Verification items for the finished model (mm, model axes). A direction names the side the tool comes from. Give positions to 0.01 mm unless a question says otherwise; leave off trailing zeros. Write each loop counter-clockwise with the first axis right and the second up, starting at its lowest first coordinate (ties: lowest second). Pieces come first, ordered by that corner, then holes. Notation, with made-up numbers: (-0.5, 3.25) -> (31.5, 3.25) arc R34 cw to (31.5, 40.25) -> close; hole circle Ø10 at (75.5, 13). An arc over 180 degrees is marked (long way). Answer as CSV lines item,"result". Start each with the question number.
1) Sectioned sample at D-D on y = 15.5. Record the cut outline in (x, z), and give its area (3 significant figures).
2) Gauge pin test, flat ends, axial feed: pin 1 Ø2 at (x, z) = (4, 9) entering from -Y; pin 2 Ø1.8 at (y, z) = (18, 6) entering from +X; pin 3 Ø1 at (x, z) = (1, 8.5) entering from -Y. Record the tip position at first contact, or that the pin passes through.
3) Sectioned sample at C-C on z = 8.75. Record the cut outline in (x, y) (3 decimals), and give its area (3 significant figures).
4) Sectioned sample at B-B on y = 34. Record the cut outline in (x, z).
5) Tool access check on faces 1 (the flat face through (3, 15, 5)), 2 (the flat face through (0, 5, 5)), 3 (the cylindrical face through (1.1, 38.3, 9)), 4 (the flat face through (0, 25, 5)). Record the directions out of +Z, -Z, +X, -X, +Y, -Y that give a thin tool (end or side, any length) a straight path to the whole face; none if there is none.
6) Mould release check, pull along Z, two halves, no side actions. Record for faces 5 (the flat face through (-3, 15, 5)), 6 (the flat face through (5, 20, 9)), 7 (the flat face through (-3.4, 20.4, 2)), 8 (the flat face through (0, 20, 0)): released by +Z, released by -Z, zero draft, split by the parting line, or undercut.
7) Material ranges on L1, parallel to Y at x = 0, z = 9.65 (3 decimals); L2, parallel to X at y = 0, z = 8.85; L3, parallel to Z at x = -3.5, y = 12, recorded low to high.
8) Sectioned sample at A-A on x = 0. Record the cut outline in (y, z) (3 decimals), and give its area (3 significant figures).
Autodesk Inventor part; units mm, degrees
ref_plane "YZ Plane" through (0, 0, 0) normal (1, 0, 0) x (0, 1, 0)
ref_plane "XZ Plane" through (0, 0, 0) normal (0, 1, 0) x (-1, 0, 0)
ref_plane "XY Plane" through (0, 0, 0) normal (0, 0, 1) x (1, 0, 0)
sketch "Sketch1" plane through (0, 0, 0) normal (0, 0, 1) x (1, 0, 0)
  circle A0 centre (0, 0) radius 2.05
  arc A1 (-5, 0) -> (5, 0) centre (0, 0) ccw
  circle A2 centre (0, 40) radius 2.025
  arc A3 (5, 40) -> (-5, 40) centre (0, 40) ccw
  line L0 (-5, 40) -> (-5, 0)
  line L1 (5, 40) -> (5, 0)
  line L2 (0, 0) -> (0, 2.05)
  line L3 (0, 37.975) -> (0, 40)
  dimension "d0" = 4.1
  dimension "d3" = 4.05
  dimension "d1" = 10
  dimension "d2" = 40
  dimension "d4" = 10
extrude "Extrusion1" add sketch "Sketch1" along normal blind 10
shell "Shell1" thickness 2 removed faces 4 at (3.9972, 43.0037, 6.6667) at (-4.9838, -0.4023, 6.6667) at (-5, 13.3333, 3.3333) at (5, 26.6667, 3.3333)
sketch "Sketch2" plane through (0, 40, 8) normal (0, 0, -1) x (-1, 0, 0)
  line L0 (-3, -35) -> (3, -35)
  line L1 (3, -35) -> (3, -15)
  line L2 (3, -15) -> (-3, -15)
  line L3 (-3, -15) -> (-3, -35)
  circle A0 centre (0, 0) radius 2.025
  point P0 (0, -40)
  dimension "d13" = 6
  dimension "d14" = 20
  dimension "d18" = 5
extrude "Extrusion2" add sketch "Sketch2" along normal blind 6 contours L3 L2 L1 L0
delete faces "Delete Face1" heal yes whole lump no faces at (4.0369, 0.3259, 4)
delete faces "Delete Face2" heal yes whole lump no faces at (4.0119, 40.3239, 4)
properties part number "Crank" material "Steel, Mild"
Ans:
1,outline,"(-5, 0) -> (5, 0) -> (5, 2) -> (3, 2) -> (3, 8) -> (5, 8) -> (5, 10) -> (-5, 10) -> (-5, 8) -> (-3, 8) -> (-3, 2) -> (-5, 2) -> close"
1,area,"76.0 mm²"
2,pin 1,"stops at y = -4"
2,pin 2,"stops at x = 3"
2,pin 3,"stops at y = -4.97"
3,outline,"(-5, 0) arc R5 ccw to (5, 0) -> (5, 40) arc R5 ccw to (-5, 40) -> close; hole circle Ø4.1 at (0, 0); hole circle Ø4.05 at (0, 40)"
3,area,"452 mm²"
4,outline,"(-5, 0) -> (5, 0) -> (5, 2) -> (-5, 2) -> close; (-5, 8) -> (5, 8) -> (5, 10) -> (-5, 10) -> close"
5,face 1,"+X, +Y, -Y"
5,face 2,"+X, -X, -Y"
5,face 3,"+Z, -Z"
5,face 4,"+X, -X, +Y"
6,face 5,"undercut"
6,face 6,"zero draft"
6,face 7,"undercut"
6,face 8,"released by -Z"
7,L1,"y = -5 to -2.05, 2.05 to 37.975, 42.025 to 45"
7,L2,"x = -5 to -2.05, 2.05 to 5"
7,L3,"z = 0 to 2, 8 to 10"
8,outline,"(-5, 0) -> (-2.05, 0) -> (-2.05, 2) -> (-5, 2) -> close; (-5, 8) -> (-2.05, 8) -> (-2.05, 10) -> (-5, 10) -> close; (2.05, 0) -> (37.975, 0) -> (37.975, 2) -> (25, 2) -> (25, 8) -> (37.975, 8) -> (37.975, 10) -> (2.05, 10) -> (2.05, 8) -> (5, 8) -> (5, 2) -> (2.05, 2) -> close; (42.025, 0) -> (45, 0) -> (45, 2) -> (42.025, 2) -> close; (42.025, 8) -> (45, 8) -> (45, 10) -> (42.025, 10) -> close"
8,area,"287 mm²"
